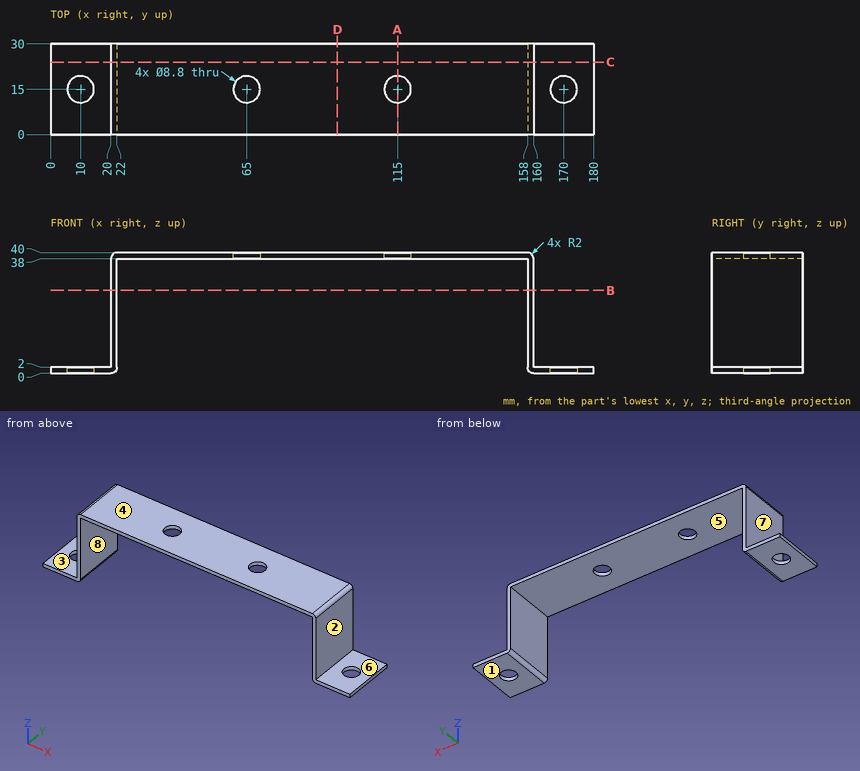
Part print with two shaded views. Sizes in mm from the minimum x, y, z corner. A direction names the side the tool comes from. Round coordinates to 2 decimals unless told otherwise and drop trailing zeros. Order: outer loops, then holes, each group sorted by start corner. A loop starts at its lowest first (then second) coordinate and runs counter-clockwise, first axis right, second up. Notation, with made-up numbers: M -38,12 L -10,12 A31 ccw -10,48 Z; hole C 71.5,89.25 d8. An arc over 180 degrees is marked long. Use CSV: the item, a comma, the result in double quotes. Start each with the question number.
(1) Cut at B-B on z = 27.5. List the corners of the cut face in (x, y).
(2) Cut at C-C on y = 24. List the corners of the cut face in (x, z), then the cut area to 3 significant figures.
(3) Tool access for the marked faces 1, 2, 3, 4 and 5: list every direction of +Z, -Z, +X, -X, +Y, -Y with a clear straight run to the whole face (end or side of a thin tool).
(4) Cut at D-D on x = 95. List the corners of the cut face in (y, z).
(5) Drill centre lines: probe 1 along Y at (x, z) = (170, 1.6); probe 2 along X at (y, z) = (11.75, 3); probe 3 along Z at (x, y) = (172.5, 5.5). Where is each one in solid material? Low to high.
(6) Flat gauge pins, fed straight in: P1, Ø11.5, axis at x = 115, y = 15, coming from the -Z side; P2, Ø10, axis at x = 11.5, y = 16, coming from the +Z side; P3, Ø3, axis at y = 3.5, z = 27, coming from the +X side. Where does each tip first touch, or does it go through?
(7) Mould opens along X. For the marked faces 6, 7 and 8 say: +X half, -X half, draft (parallel to the pull), parting line (faces both ways), or undercut.
(8) Cut at A-A on x = 115. List the corners of the cut face in (y, z).
Findings:
1,outline,"M 20,0 L 22,0 L 22,30 L 20,30 Z; M 158,0 L 160,0 L 160,30 L 158,30 Z"
2,outline,"M 0,0 L 20,0 A2 ccw 22,2 L 22,38 L 158,38 L 158,2 A2 ccw 160,0 L 180,0 L 180,2 L 160,2 L 160,38 A2 ccw 158,40 L 22,40 A2 ccw 20,38 L 20,2 L 0,2 Z"
2,area,"509 mm^2"
3,face 1,"-Z, +X, -X, +Y, -Y"
3,face 2,"+Z, +X, +Y, -Y"
3,face 3,"+Z, -X, +Y, -Y"
3,face 4,"+Z, +X, -X, +Y, -Y"
3,face 5,"-Z, +Y, -Y"
4,outline,"M 0,38 L 30,38 L 30,40 L 0,40 Z"
5,probe 1,"y = 0 to 10.6, 19.4 to 30"
5,probe 2,"x = 20 to 22, 158 to 160"
5,probe 3,"z = 0 to 2"
6,P1,"stops at z = 38"
6,P2,"stops at z = 2"
6,P3,"stops at x = 160"
7,face 6,"draft"
7,face 7,"-X half"
7,face 8,"undercut"
8,outline,"M 0,38 L 10.6,38 L 10.6,40 L 0,40 Z; M 19.4,38 L 30,38 L 30,40 L 19.4,40 Z"
